from build123d import *

# Parameters (mm, degrees)
SKETCH3_R   = 16.764
SKETCH3_R_2 = 12.6873


with BuildPart() as part:
    # Sketch1 → Revolve1 (revolve)
    with BuildSketch(Plane.XY, mode=Mode.PRIVATE) as revolve1_sk:
        Polygon((-14.732, -12.6873), (-14.732, -16.764), (-35.56, -16.764), (-35.56, -13.335), align=None)
    revolve(revolve1_sk.sketch.rotate(Axis((-35.56, 0, 0), (1, 0, 0)), 270), axis=Axis((-35.56, 0, 0), (1, 0, 0)))


with BuildPart() as body_2:
    # Sketch2 → Revolve2 (revolve)
    with BuildSketch(Plane.XY, mode=Mode.PRIVATE) as revolve2_sk:
        Polygon((13.335, 35.56), (12.686518, 14.732), (16.764, 14.732), (16.764, 35.56), align=None)
    revolve(revolve2_sk.sketch.rotate(Axis((0, 0, 0), (0, 1, 0)), 90), axis=Axis((0, 0, 0), (0, 1, 0)))


with BuildPart() as sweep1_tool:
    # Sweep1: sweep along a path in Sketch4
    with BuildLine(Plane.XY) as sweep1_path:
        ThreePointArc((-14.732, 0), (-4.314903, 4.314903), (0, 14.732))
    # Sketch3 → Sweep1 (sweep)
    with BuildSketch(Plane(origin=(-14.732, 0, 0), x_dir=(0, 0, -1), z_dir=(1, 0, 0))):
        Circle(SKETCH3_R)
        Circle(SKETCH3_R_2, mode=Mode.SUBTRACT)
    sweep(path=sweep1_path.line)


with BuildPart() as part_1:
    add(part.part)


with BuildPart() as part_2:
    # Sweep1: joined with sweep1_tool
    add(part_1.part.fuse(sweep1_tool.part, body_2.part, tol=0.00001))


solid = part_2.part
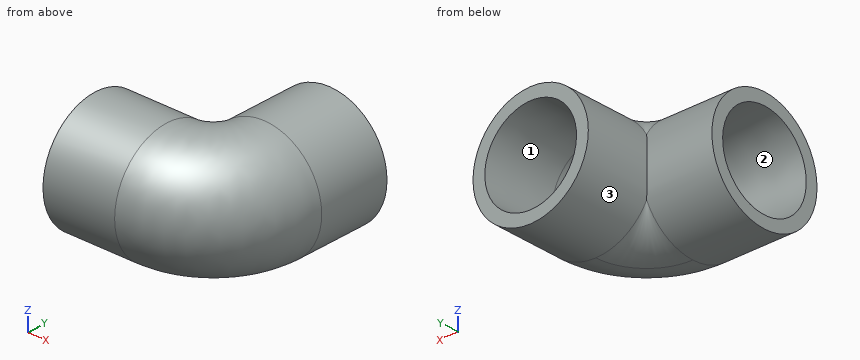
Work out the finished part from the listing and answer in its coordinate system (mm). Face numbers are marked on the shaded views. Give positions to 0.01 mm unless a question says otherwise; leave off trailing zeros. Order: outer loops, then holes, each group sorted by start corner. A loop starts at its lowest first (then second) coordinate and runs counter-clockwise, first axis right, second up. Notation, with made-up numbers: (-20, 7) -> (-13, 7) arc R13 ccw to (-13, 18) -> close; hole circle Ø11 at (29.5, -9). An arc over 180 degrees is marked (long way). Answer as a JSON object with one key per item and string values. Group by question number.
1. Section A-A on x = -16 is taken. Determine the outline of the cut face in (y, z).
2. Flat-ended cylindrical pins translate along their axes: pin 1 Ø7.5 at (x, z) = (6, -3.5) entering from -Y; pin 2 Ø1 at (x, y) = (-5.5, -4) entering from -Z; pin 3 Ø12 at (x, z) = (-19, 10.5) entering from -Y; pin 4 Ø8 at (x, y) = (-24.5, -1) entering from +Z. Find the tip coordinate at first contact, or state that the pin passes through.
3. Consider line 1 along Z through (x, y) = (-5.5, 4.5); line 2 along X through (y, z) = (22, -4); line 3 along X through (y, z) = (20.5, 8.5). Determine where each line is inside the solid, lowest interval first. Write a range as [from, to].
4. The mould has two halves that part along Y. Classify the marked faces 1, 2 and 3: released by +Y, released by -Y, zero draft, split by the parting line, or undercut.
Result sheet:
{
 "1": {"outline": "(16, -5) -> (35.56, -5) -> (35.56, 5) -> (16, 5) arc R16.76 ccw (long way) to start; hole circle Ø25.45 at (0, 0)"},
 "2": {"pin 1": "stops at y = -11.48", "pin 2": "stops at z = -15.78", "pin 3": "stops at y = -16.15", "pin 4": "stops at z = 16.76"},
 "3": {"line 1": "z = [-16.74, -12.65], [12.65, 16.74]", "line 2": "x = [-16.28, -12.28], [12.28, 16.28]", "line 3": "x = [-14.45, -9.66], [9.66, 14.45]"},
 "4": {"face 1": "released by +Y", "face 2": "undercut", "face 3": "zero draft"}
}
